Here's how the part is built. I have some questions about the finished solid (model axes, mm). A direction names the side the tool comes from. Coordinates: 2 decimals unless noted, no trailing zeros. Write each loop counter-clockwise with the first axis right and the second up, starting at its lowest first coordinate (ties: lowest second). Pieces come first, ordered by that corner, then holes. Notation, with made-up numbers: (38, 87.5) -> (82, 87.5) arc R13 cw to (82, 111.5) -> close; hole circle Ø3 at (19, 39). An arc over 180 degrees is marked (long way). Use a Markdown table: item, result. Add a question column.
```python
from build123d import *

# Parameters (mm, degrees)
BOSS_EXTRUDE1_DEPTH = 228.6
FILLET1_R           = 2.54


with BuildPart() as part:
    # Sketch1 → Boss-Extrude1 (new, symmetric)
    with BuildSketch(Plane.XY):
        with BuildLine():
            Line((0, 0), (25.4, 0))
            Line((25.4, 0), (25.4, 3.175))
            Line((25.4, 3.175), (4.445, 3.175))
            ThreePointArc((4.445, 3.175), (3.546974388, 3.546974388), (3.175, 4.445))
            Line((3.175, 4.445), (3.175, 25.400000027))
            Line((3.175, 25.400000027), (0, 25.400000027))
            Line((0, 25.400000027), (0, 0))
        make_face()
    extrude(amount=BOSS_EXTRUDE1_DEPTH, both=True)

    # Sketch3 → CSK for #10 Flat Head Machine Screw1 (revolve, cut)
    with BuildSketch(Plane(origin=(15.875, 0, -203.2), x_dir=(0, 0, -1), z_dir=(1, 0, 0))):
        Polygon((0, 0), (0, 3.175), (2.4892, 3.175), (2.4892, 2.761229288), (4.8895, 0), align=None)
    csk_for_10_flat_head_machine_screw1 = revolve(axis=Axis((15.875, -6.35, -203.2), (0, 1, 0)), mode=Mode.SUBTRACT)

    # Mirror1: CSK for #10 Flat Head Machine Screw1 across plane
    add(csk_for_10_flat_head_machine_screw1.mirror(Plane.XY), mode=Mode.SUBTRACT)

    # Fillet1
    fillet1_edges = [part.edges().sort_by_distance(p)[0] for p in [
        (25.4, 1.5875, 228.6),
        (1.5875, 25.400000027, 228.6),
        (1.5875, 25.400000027, -228.6),
        (25.4, 1.5875, -228.6),
    ]]
    fillet(fillet1_edges, radius=FILLET1_R)


solid = part.part
```
Q1. Please list where these lines run through material, in increasing order: line 1 (X direction, y = 3, z = 203.2); line 2 (X direction, y = 16, z = -138.5) (3 decimals).
Q2. Thinking about a two-plate mould opening in Z: for faces 1 (the flat face through (3, 7, 228.6)), 2 (the conical face through (15.759, 2.588, -200.563)), 3 (the flat face through (15, 3.175, 3)), 4 (the flat face through (3, 7, -228.6)), which applies, released by +Z, released by -Z, zero draft, split by the parting line, or undercut?
Q3. Suppose I cut it at A-A, the plane z = -176.5. Write out the boundary of the cut face in (x, y) (3 decimals).
Q4. Will these pins go through, and if not, where does the flat tip stop? pin 1 (8 mm diameter, centred on x = 13.5, z = 122, fed in from -Y); pin 2 (5.5 mm diameter, centred on x = 15.875, z = -203.2, fed in from -Y); pin 3 (10.5 mm diameter, centred on y = 12.5, z = 28, fed in from +X) (3 decimals); pin 4 (3 mm diameter, centred on x = 5.5, z = -141.5, fed in from +Y).
Q5. Which directions (+Z, -Z, +X, -X, +Y, -Y) give clear straight access to the entire face, cutting with the end or side of a thin tool? Please do faces 5 (the conical face through (15.759, 2.588, 200.563)), 6 (the flat face through (3.175, 15, 3)).
Answer key:
| question | item | result |
|---|---|---|
| 1 | line 1 | x = 0 to 13.39, 18.36 to 25.4 |
| 1 | line 2 | x = 0 to 3.175 |
| 2 | face 1 | released by +Z |
| 2 | face 2 | undercut |
| 2 | face 3 | zero draft |
| 2 | face 4 | released by -Z |
| 3 | outline | (0, 0) -> (25.4, 0) -> (25.4, 3.175) -> (4.445, 3.175) arc R1.27 cw to (3.175, 4.445) -> (3.175, 25.4) -> (0, 25.4) -> close |
| 4 | pin 1 | stops at y = 0 |
| 4 | pin 2 | stops at y = 2.46 |
| 4 | pin 3 | stops at x = 3.175 |
| 4 | pin 4 | stops at y = 3.26 |
| 5 | face 5 | -Y |
| 5 | face 6 | +Z, -Z, +X, +Y |
